Autodesk Inventor part; units mm, degrees
ref_plane "YZ Plane" through (0, 0, 0) normal (1, 0, 0) x (0, 1, 0)
ref_plane "XZ Plane" through (0, 0, 0) normal (0, 1, 0) x (-1, 0, 0)
ref_plane "XY Plane" through (0, 0, 0) normal (0, 0, 1) x (1, 0, 0)
sketch "스케치1" plane through (0, 0, 0) normal (1, 0, 0) x (0, 1, 0)
  line L0 (0, 0) -> (4, 0)
  line L1 (4, 0) -> (4, 10)
  line L2 (4, 10) -> (0, 10)
  line L3 (0, 10) -> (0, 0)
  line L4 (0, 10) -> (5, 10)
  line L5 (5, 10) -> (5, 33)
  line L6 (5, 33) -> (0, 33)
  line L7 (0, 33) -> (0, 10)
  line L8 (0, 33) -> (6, 33)
  line L9 (6, 33) -> (6, 53)
  line L10 (6, 53) -> (0, 53)
  line L11 (0, 53) -> (0, 33)
  line L12 (0, 53) -> (8, 53)
  line L13 (8, 53) -> (8, 153)
  line L14 (8, 153) -> (0, 153)
  line L15 (0, 153) -> (0, 53)
  dimension "d0" = 100
  dimension "d1" = 20
  dimension "d2" = 23
  dimension "d3" = 10
  dimension "d4" = 8
  dimension "d5" = 10
  dimension "d6" = 12
  dimension "d7" = 16
revolve "회전1" add sketch "스케치1" angle 360 about axis through (0, 0, 33) along (0, 0, -1)
thread "스레드1"
sketch "스케치2" plane through (0, 0, 0) normal (1, 0, 0) x (0, 1, 0)
  line L0 (6, 53) -> (6, 33)
  line L1 (-6, 33) -> (6, 33)
  line L2 (6, 33) -> (6, 34.5588)
  line L3 (6, 33) -> (5.1, 33)
  line L4 (5.1, 33) -> (6, 34.5588)
  line L5 (0, -30.6) -> (0, 183.6)
  point P0 (0, 0)
  dimension "d11" = 0.9
  dimension "d12" = 30
revolve "회전2" cut sketch "스케치2" angle 360 about axis through (0, 0, -10) along (0, 0, 1)
fillet "모깎기1" radius 4 1 edges at (0, -6, 34.5588)
fillet "모깎기2" radius 1 1 edges at (0, -5.1, 33)
sketch "스케치3" plane through (0, 0, 0) normal (1, 0, 0) x (0, 1, 0)
  line L0 (5, 33) -> (5, 10)
  line L1 (5, 14) -> (3.2, 14)
  line L2 (3.2, 14) -> (3.2, 24)
  line L3 (3.2, 24) -> (5, 24)
  line L4 (5, 24) -> (5, 14)
  point P0 (0, 0)
  dimension "d16" = 1.8
  dimension "d17" = 10
  dimension "d18" = 4
extrude "돌출1" cut sketch "스케치3" along normal mid plane 3
fillet "모깎기3" radius 1.5 4 edges at (1.5, 3.9848, 14) (-1.5, 3.9848, 14) (-1.5, 3.9848, 24) (1.5, 3.9848, 24)
chamfer "모따기1" distance 1 angle 45 2 edges at (0, -8, 153) (0, -4, 0)
sketch "스케치4" plane through (0, 0, 0) normal (1, 0, 0) x (0, 1, 0)
  line L0 (4, 10) -> (4, 6.25)
  line L1 (4, 6.25) -> (3, 8)
  line L2 (3, 8) -> (3, 10)
  line L3 (3, 10) -> (4, 10)
  line L4 (-5, 10) -> (5, 10)
  line L5 (0, -30.6) -> (0, 183.6)
  point P0 (0, 0)
  dimension "d25" = 1
  dimension "d26" = 2
  dimension "d27" = 3.75
revolve "회전3" cut sketch "스케치4" angle 360 about axis through (0, 0, -10) along (0, 0, 1)
fillet "모깎기4" radius 0.6 2 edges at (0, -3, 8) (0, -3, 10)
properties part number "도면1-2번"
For this review, take the finished solid that the model builds, in its own axes (mm). A direction names the side the tool comes from. Give positions to 0.01 mm unless a question says otherwise; leave off trailing zeros. Write each loop counter-clockwise with the first axis right and the second up, starting at its lowest first coordinate (ties: lowest second). Pieces come first, ordered by that corner, then holes.
Item 1: The part is to be moulded in two halves that separate along Z. For faces 1 (the face through (0, 0, 0)), 2 (the face through (0, -3, 9)), 3 (the face through (0, 3.2, 19)), 4 (the face through (0, 0, 153)), say which applies: +Z half, -Z half, draft (parallel to the pull), parting line (faces both ways), or undercut.
Item 2: Machinability: for faces 5 (the face through (7.81, -1.73, 103.19)), 6 (the face through (2.2, 3.3, 10)), 7 (the face through (6, -2, 53)), which of the approach directions +Z, -Z, +X, -X, +Y, -Y give a long, thin tool a straight path to every point of the face, cutting with its end or side? Answer none if there is none.
Item 3: Insertion check: P1, Ø1, axis at x = 6, z = 95, coming from the +Y side; P2, Ø5, axis at x = -3, z = 91, coming from the -Y side; P3, Ø0.5, axis at y = 4, z = 18.5, coming from the +X side; P4, Ø5, axis at x = -2, y = -2.5, coming from the -Z side. Each pin has a flat end and moves straight along its axis. Give the tip position at first contact, or say it passes through.
Item 4: Wall thickness on probe 1 along Z at (x, y) = (-4, -5.5); probe 2 along Z at (x, y) = (5.25, -1.5); probe 3 along Y at (x, z) = (-0.5, 80.5): over which ranges is each line inside the solid? List them lowest first.
Item 5: Take a section at A-A (z = 90). Give the boundary of the cut face in (x, y), and give its area (3 significant figures).
Established:
1. face 1: -Z half
1. face 2: undercut
1. face 3: undercut
1. face 4: +Z half
2. face 5: +Z, -Z
2. face 6: none
2. face 7: -Z
3. P1: stops at y = 5.81
3. P2: stops at y = -7.98
3. P3: stops at x = 3.31
3. P4: stops at z = 0
4. probe 1: z = 53 to 153
4. probe 2: z = 33.62 to 153
4. probe 3: y = -7.98 to 7.98
5. outline: circle Ø16 at (0, 0)
5. area: 201 mm2
